Can you work these out from the model? Positions are in its coordinate system, mm. A direction names the side the tool comes from. Give positions to 0.01 mm unless a question says otherwise; leave off trailing zeros. Order: outer loops, then holes, each group sorted by start corner. A loop starts at its lowest first (then second) coordinate and runs counter-clockwise, first axis right, second up. Notation, with made-up numbers: (-27.5, 6) -> (23.5, 6) arc R25 cw to (23.5, 26) -> close; hole circle Ø5 at (74, 62). An arc over 180 degrees is marked (long way). Answer as a JSON object with one key per item and string values.
```python
from build123d import *

# Parameters (mm, degrees)
SKETCH1_W           = 11.049
SKETCH1_H           = 26.9875
BOSS_EXTRUDE1_DEPTH = 1.5875
SKETCH2_W           = 7.874
SKETCH2_H           = 1.5875
BOSS_EXTRUDE2_DEPTH = 2.794
CUT_EXTRUDE1_REACH  = 6.381
SKETCH3_R           = 0.3175


with BuildPart() as part:
    # Sketch1 → Boss-Extrude1 (new body)
    with BuildSketch(Plane(origin=(0, 0, 0), x_dir=(0, 0, -1), z_dir=(1, 0, 0))):
        Rectangle(SKETCH1_W, SKETCH1_H)
    extrude(amount=BOSS_EXTRUDE1_DEPTH)

    # Sketch2 → Boss-Extrude2 (add)
    with BuildSketch(Plane(origin=(1.5875, 0, 0), x_dir=(0, 0, -1), z_dir=(1, 0, 0))):
        with Locations((0, 12.7)):
            Rectangle(SKETCH2_W, SKETCH2_H)
    extrude(amount=BOSS_EXTRUDE2_DEPTH)

    # Sketch3 → Cut-Extrude1 (cut, up to next)
    with BuildSketch(Plane.ZY, mode=Mode.PRIVATE) as cut_extrude1_sk1:
        with Locations((-2.3495, 1.74625)):
            Circle(SKETCH3_R)
    cut_extrude1_tool1 = extrude(cut_extrude1_sk1.sketch, amount=-CUT_EXTRUDE1_REACH, mode=Mode.PRIVATE) & part.part
    add(cut_extrude1_tool1.solids().sort_by_distance((0, 1.74625, -2.3495))[0], mode=Mode.SUBTRACT)
    # Sketch3 → Cut-Extrude1 (cut, up to next)
    with BuildSketch(Plane.ZY, mode=Mode.PRIVATE) as cut_extrude1_sk2:
        with Locations((-2.3495, -9.68375)):
            Circle(SKETCH3_R)
    cut_extrude1_tool2 = extrude(cut_extrude1_sk2.sketch, amount=-CUT_EXTRUDE1_REACH, mode=Mode.PRIVATE) & part.part
    add(cut_extrude1_tool2.solids().sort_by_distance((0, -9.68375, -2.3495))[0], mode=Mode.SUBTRACT)


solid = part.part
```
1. If we section it at C-C on y = 9.5: Please give me the cut outline in (x, z), then the cut area to 3 significant figures.
Worked answers:
{"outline": "(0, -5.52) -> (1.59, -5.52) -> (1.59, 5.52) -> (0, 5.52) -> close", "area": "17.5 mm²"}
2. If we section it at B-B on x = 3.15: Please give me the cut outline in (y, z).
Worked answers:
{"outline": "(11.91, -3.94) -> (13.49, -3.94) -> (13.49, 3.94) -> (11.91, 3.94) -> close"}
3. If we section it at A-A on z = 3: Please give me the cut outline in (x, y).
Worked answers:
{"outline": "(0, -13.49) -> (1.59, -13.49) -> (1.59, 11.91) -> (4.38, 11.91) -> (4.38, 13.49) -> (0, 13.49) -> close"}
4. For faces 1 (the face through (3, 11.906, 0)), 2 (the face through (3, 13, -3.937)), 3 (the face through (3, 13, 3.937)), 4 (the face through (2, 13.494, 0)), which set-ups out of +Z, -Z, +X, -X, +Y, -Y let a thin tool reach every point of the face, with its end or its side?
Worked answers:
{"face 1": "+Z, -Z, +X, -Y", "face 2": "-Z, +X, +Y, -Y", "face 3": "+Z, +X, +Y, -Y", "face 4": "+Z, -Z, +X, -X, +Y"}
5. Will these pins go through, and if not, where does the flat tip stop? pin 1 Ø1.5 at (y, z) = (2, -2) entering from +X; pin 2 Ø1.3 at (x, y) = (3, 13) entering from +Z; pin 3 Ø1.7 at (x, y) = (3, 13) entering from -Z.
Worked answers:
{"pin 1": "x = 1.59", "pin 2": "z = 3.94", "pin 3": "z = -3.94"}
6. Please list where these lines run through material, in increasing order: L1, parallel to X at y = -9.75, z = 1.5; L2, parallel to Y at x = 2.5, z = 2; L3, parallel to Z at x = 0.65, y = -9.5.
Worked answers:
{"L1": "0 to 1.59", "L2": "11.91 to 13.49", "L3": "-5.52 to -2.61, -2.09 to 5.52"}
